from build123d import *

# Parameters (mm, degrees)
CUT_EXTRUDE1_DEPTH = 8.9
SKETCH3_W          = 20
SKETCH3_H          = 20
CUT_EXTRUDE2_DEPTH = 2


with BuildPart() as part:
    # Sketch1 → Revolve1 (revolve)
    with BuildSketch(Plane(origin=(0, 0, 0), x_dir=(0, 0, -1), z_dir=(1, 0, 0))):
        with BuildLine():
            Line((-3.4, 0), (-3.4, 3))
            Line((-3.4, 3), (-15.1, 3))
            ThreePointArc((-15.1, 3), (-15.312132034, 3.087867966), (-15.4, 3.3))
            Line((-15.4, 3.3), (-14.970691475, 5.734729636))
            ThreePointArc((-14.970691475, 5.734729636), (-14.902287446, 5.853208889), (-14.773729924, 5.9))
            Line((-14.773729924, 5.9), (-13.6, 5.9))
            Line((-13.6, 5.9), (-13.6, 4.075))
            ThreePointArc((-13.6, 4.075), (-13.490165043, 3.809834957), (-13.225, 3.7))
            Line((-13.225, 3.7), (-12.8, 3.7))
            Line((-12.8, 3.7), (-12.8, 4.729289322))
            Line((-12.8, 4.729289322), (-12.729289322, 4.8))
            Line((-12.729289322, 4.8), (-12.5, 4.8))
            Line((-12.5, 4.8), (-12.5, 4.9))
            Line((-12.5, 4.9), (-0.7, 4.9))
            Line((-0.7, 4.9), (-0.7, 4.8))
            Line((-0.7, 4.8), (-0.6, 4.8))
            Line((-0.6, 4.8), (-0.5, 4.7))
            Line((-0.5, 4.7), (-0.4, 4.8))
            Line((-0.4, 4.8), (0, 4.8))
            Line((0, 4.8), (0, 3.5))
            Line((0, 3.5), (4.8865, 3.5))
            Line((4.8865, 3.5), (5.5, 2.8865))
            Line((5.5, 2.8865), (5.5, 0))
            Line((5.5, 0), (-3.4, 0))
        make_face()
    revolve(axis=Axis((0, 0, -5.5), (0, 0, 1)))

    # Sketch2 → Cut-Extrude1 (cut)
    with BuildSketch(Plane.XY.offset(-5.5)):
        Polygon((-2, -1.154700538), (0, -2.309401077), (2, -1.154700538), (2, 1.154700538), (0, 2.309401077), (-2, 1.154700538), align=None)
    extrude(amount=CUT_EXTRUDE1_DEPTH, mode=Mode.SUBTRACT)

    # Sketch3 → Cut-Extrude2 (cut)
    with BuildSketch(Plane.XY.offset(15.4)):
        Rectangle(SKETCH3_W, SKETCH3_H)
        with BuildLine():
            Line((-4.9, 1), (-4.9, -0.999999812))
            ThreePointArc((-4.9, -0.999999812), (0, -5.899999812), (4.9, -0.999999812))
            Line((4.9, -0.999999812), (4.9, 1))
            ThreePointArc((4.9, 1), (0, 5.9), (-4.9, 1))
        make_face(mode=Mode.SUBTRACT)
    extrude(amount=-CUT_EXTRUDE2_DEPTH, mode=Mode.SUBTRACT)


solid = part.part
The model under review builds one solid part; all positions refer to its coordinate system, in mm. A direction names the side the tool comes from. Round coordinates to 2 decimals unless told otherwise and drop trailing zeros. Loops run counter-clockwise (first coordinate to the right, second up) from the corner with the lowest first, then second, coordinate; pieces in that order, holes last. Notation, with made-up numbers: (67.5, -2) -> (114.5, -2) arc R33 ccw to (114.5, 30) -> close; hole circle Ø9 at (36, 48). An arc over 180 degrees is marked (long way). Return JSON: item names as keys, results as strings.
(1) For line 1 (X direction, y = 0, z = 10.75); line 2 (Y direction, x = 0, z = 12.75), list the stretches that pass through material, from the lowest coordinate up.
Solved:
{"line 1": "-4.9 to -3, 3 to 4.9", "line 2": "-4.78 to -3, 3 to 4.78"}
(2) Add section B-B on z = 5. Write out the cut boundary in (x, y).
Solved:
{"outline": "circle Ø9.8 at (0, 0); hole circle Ø6 at (0, 0)"}
(3) Add section A-A on z = 1.5. Write out the cut boundary in (x, y).
Solved:
{"outline": "circle Ø9.8 at (0, 0); hole (-2, -1.15) -> (0, -2.31) -> (2, -1.15) -> (2, 1.15) -> (0, 2.31) -> (-2, 1.15) -> close"}
(4) For pin 1 (2 mm diameter, centred on x = 1, z = -3, fed in from -Y); pin 2 (1 mm diameter, centred on x = 2, y = 4, fed in from -Z); pin 3 (3 mm diameter, centred on x = -2.5, z = -3.5, fed in from +Y), all flat-tipped, find the tip position at first contact; note any pin that passes through.
Solved:
{"pin 1": "y = -3.5", "pin 2": "z = 0", "pin 3": "y = 3.35"}
(5) For faces 4 (the flat face through (-0.99, 1.74, -1.11)), 5 (the flat face through (4.9, 0, 14)), 6 (the conical face through (-1.037, 3.293, 15.373)), 7 (the flat face through (4, 0, 0)), 8 (the cylindrical face through (3.612, -0.802, 13.01)), list the 3-axis set-ups (+Z, -Z, +X, -X, +Y, -Y) from which the entire face can be reached by the end or side of a thin tool; tool diameter is ignored.
Solved:
{"face 4": "+Z, -Z", "face 5": "+Z, -Z, +X, +Y, -Y", "face 6": "+Z", "face 7": "-Z", "face 8": "none"}
(6) The part is to be moulded in two halves that separate along Z. For faces 1 (the flat face through (3, -3, 13.6)), 2 (the flat face through (1, -2, -5.5)), 3 (the cylindrical face through (0, -3, 9)), say which applies: released by +Z, released by -Z, zero draft, split by the parting line, or undercut.
Solved:
{"face 1": "undercut", "face 2": "released by -Z", "face 3": "zero draft"}
